The listing builds one solid part. Answer for the finished solid, in the listing's coordinates (mm). A direction names the side the tool comes from. Coordinates: 2 decimals unless noted, no trailing zeros. Order: outer loops, then holes, each group sorted by start corner. A loop starts at its lowest first (then second) coordinate and runs counter-clockwise, first axis right, second up.
from build123d import *

# Parameters (mm, degrees)
BOSS_EXTRU_2_DEPTH      = 2
BOSS_EXTRU_3_DEPTH      = 2
ESQUISSE4_R             = 0.5
ENL_V_MAT_EXTRU_1_DEPTH = 2
ESQUISSE5_R             = 0.2
ENL_V_MAT_EXTRU_2_DEPTH = 1
ESQUISSE6_R             = 0.2
ENL_V_MAT_EXTRU_3_DEPTH = 1
CHANFREIN1_SIZE         = 0.2
CHANFREIN2_SIZE         = 0.2
CHANFREIN3_SIZE         = 0.2


with BuildPart() as part:
    # Esquisse1 → Boss.-Extru.2 (new body)
    with BuildSketch(Plane.XY):
        Polygon((-4.954240171, 0), (-0.954240171, 0), (-0.954240171, 1), (-1.954240171, 1), (-1.954240171, 6), (-3.954240171, 6), (-3.954240171, 1), (-4.954240171, 1), align=None)
    extrude(amount=BOSS_EXTRU_2_DEPTH)

    # Esquisse3 → Boss.-Extru.3 (add)
    with BuildSketch(Plane.XY.offset(2)):
        Polygon((-3.954240171, 1), (-1.954240171, 1), (-0.954240171, 1), (-0.954240171, 0), (-4.954240171, 0), (-4.954240171, 1), align=None)
    extrude(amount=BOSS_EXTRU_3_DEPTH)

    # Esquisse4 → Enlèv. mat.-Extru.1 (cut)
    with BuildSketch(Plane.XY.offset(2)):
        with Locations((-2.954240171, 5)):
            Circle(ESQUISSE4_R)
    extrude(amount=-ENL_V_MAT_EXTRU_1_DEPTH, mode=Mode.SUBTRACT)

    # Esquisse5 → Enlèv. mat.-Extru.2 (cut)
    with BuildSketch(Plane.ZY.offset(3.954240171)):
        with Locations((1, 5)):
            Circle(ESQUISSE5_R)
    extrude(amount=-ENL_V_MAT_EXTRU_2_DEPTH, mode=Mode.SUBTRACT)

    # Esquisse6 → Enlèv. mat.-Extru.3 (cut)
    with BuildSketch(Plane(origin=(0, 1, 0), x_dir=(1, 0, 0), z_dir=(0, 1, 0))):
        with Locations((-4.454240171, -1)):
            Circle(ESQUISSE6_R)
        with Locations((-1.454240171, -1)):
            Circle(ESQUISSE6_R)
        with Locations((-2.954240171, -3)):
            Circle(ESQUISSE6_R)
    extrude(amount=-ENL_V_MAT_EXTRU_3_DEPTH, mode=Mode.SUBTRACT)

    # Chanfrein1
    chanfrein1_edges = [part.edges().sort_by_distance(p)[0] for p in [
        (-3.154240171, 1, 3),
    ]]
    chamfer(chanfrein1_edges, length=CHANFREIN1_SIZE)

    # Chanfrein2
    chanfrein2_edges = [part.edges().sort_by_distance(p)[0] for p in [
        (-1.654240171, 1, 1),
    ]]
    chamfer(chanfrein2_edges, length=CHANFREIN2_SIZE)

    # Chanfrein3
    chanfrein3_edges = [part.edges().sort_by_distance(p)[0] for p in [
        (-4.654240171, 1, 1),
    ]]
    chamfer(chanfrein3_edges, length=CHANFREIN3_SIZE)


solid = part.part
1) Section A-A (z = 3) is taken. Give the vertices of the cut face in (x, y), then the cut area to 3 significant figures.
2) Section C-C (z = 1) is taken. Give the vertices of the cut face in (x, y), then the cut area to 3 significant figures.
3) Section D-D (x = -2.25) is taken. Give the vertices of the cut face in (y, z), then the cut area to 3 significant figures.
4) A tool of negligible diameter and unlimited length cuts with its end or side. For faces 1 (the face through (-3.954, 4, 1)), 2 (the face through (-3, 2, 0)), 3 (the face through (-1.954, 3, 1)), from which of +Z, -Z, +X, -X, +Y, -Y can it reach the whole face along a straight path? Write none if from no direction.
5) Each of these flat-tipped pins is pushed along its axis until it touches: P1, Ø1, axis at y = 3, z = 1, coming from the +X side; P2, Ø2, axis at x = -3, y = 3, coming from the +Z side; P3, Ø1, axis at y = 3, z = 0.5, coming from the -X side. Where does it stop, or does it pass through?
6) Section B-B (y = 5) is taken. Give the vertices of the cut face in (x, z).
7) Determine the mould class of faces 4 (the face through (-3, 0, 2)), 5 (the face through (-3, 6, 1)), 6 (the face through (-2.477, 5.15, 1.014)), 7 (the face through (-3, 4, 2)) for opening direction Y: released by +Y, released by -Y, zero draft, split by the parting line, or undercut.
8) Consider L1, parallel to X at y = 0.6, z = 1; L2, parallel to Z at x = -3.6, y = 5; L3, parallel to Y at x = -3.55, z = 1. Determine where each line is inside the solid, lowest interval first.
Filled sheet:
1. outline: (-4.95, 0) - (-3.15, 0) - (-3.15, 0.8) - (-3.35, 1) - (-4.95, 1) - close; (-2.75, 0) - (-0.95, 0) - (-0.95, 1) - (-2.55, 1) - (-2.75, 0.8) - close
1. area: 3.56 mm2
2. outline: (-4.95, 0) - (-4.65, 0) - (-4.65, 0.8) - (-4.85, 1) - (-4.95, 1) - close; (-4.25, 0) - (-1.65, 0) - (-1.65, 0.8) - (-1.85, 1) - (-1.95, 1) - (-1.95, 6) - (-3.95, 6) - (-3.95, 5.2) - (-3.41, 5.2) arc R0.5 cw (long way) to (-3.41, 4.8) - (-3.95, 4.8) - (-3.95, 1) - (-4.05, 1) - (-4.25, 0.8) - close; (-1.25, 0) - (-0.95, 0) - (-0.95, 1) - (-1.05, 1) - (-1.25, 0.8) - close
2. area: 12.1 mm2
3. outline: (0, 0) - (6, 0) - (6, 2) - (1, 2) - (1, 4) - (0, 4) - close
3. area: 14.0 mm2
4. face 1: +Z, -Z, -X, +Y
4. face 2: -Z, +X, -X, +Y, -Y
4. face 3: +Z, -Z, +X, +Y
5. P1: stops at x = -1.95
5. P2: stops at z = 2
5. P3: stops at x = -3.95
6. outline: (-3.95, 0) - (-3.45, 0) - (-3.45, 0.8) - (-3.95, 0.8) - close; (-3.95, 1.2) - (-3.45, 1.2) - (-3.45, 2) - (-3.95, 2) - close; (-2.45, 0) - (-1.95, 0) - (-1.95, 2) - (-2.45, 2) - close
7. face 4: released by -Y
7. face 5: released by +Y
7. face 6: undercut
7. face 7: zero draft
8. L1: x = -4.95 to -4.65, -4.25 to -1.65, -1.25 to -0.95
8. L2: z = 0 to 0.8, 1.2 to 2
8. L3: y = 0 to 4.8, 5.2 to 6
